```python
from build123d import *

# Parameters (mm, degrees)
SKETCH1_R           = 30
BOSS_EXTRUDE1_DEPTH = 6.35


with BuildPart() as part:
    # Sketch1 → Boss-Extrude1 (new, symmetric)
    with BuildSketch(Plane(origin=(0, 0, 0), x_dir=(0, 0, -1), z_dir=(1, 0, 0))):
        with BuildLine():
            Line((90, 0), (90, 45))
            Line((90, 45), (51.784861392, 110.303929293))
            ThreePointArc((51.784861392, 110.303929293), (0, 140), (-51.784861392, 110.303929293))
            Line((-51.784861392, 110.303929293), (-90, 45))
            Line((-90, 45), (-90, 0))
            Line((-90, 0), (90, 0))
        make_face()
        with Locations((0, 80)):
            Circle(SKETCH1_R, mode=Mode.SUBTRACT)
    extrude(amount=BOSS_EXTRUDE1_DEPTH, both=True)


solid = part.part
```
Model file for the job. Use its own axes, mm. Coordinates: 2 decimals unless noted, no trailing zeros. Order: outer loops, then holes, each group sorted by start corner. A loop starts at its lowest first (then second) coordinate and runs counter-clockwise, first axis right, second up. Notation, with made-up numbers: (13.25, 1) -> (41.25, 1) arc R15 cw to (41.25, 26) -> close; hole circle Ø8 at (81.25, 57.25). An arc over 180 degrees is marked (long way). Return JSON: item names as keys, results as strings.
Item 1: Pin check, flat tips, straight feed: P1, Ø6, axis at x = 1.5, y = 72.5, coming from the -Z side; P2, Ø1.5, axis at x = -0.5, z = -67, coming from the +Y side. Stop position of each tip, or through.
Model answer:
{"P1": "stops at z = -75.66", "P2": "stops at y = 85.59"}
Item 2: Slice it at D-D (z = -75.5). Write the cut outline in (x, y), then the cut area to 3 significant figures.
Model answer:
{"outline": "(-6.35, 0) -> (6.35, 0) -> (6.35, 69.78) -> (-6.35, 69.78) -> close", "area": "886 mm²"}
Item 3: Wall check: line 1 along Y through (x, z) = (-3.5, 0); line 2 along Y through (x, z) = (-3.25, -10.5); line 3 along Z through (x, y) = (-4.75, 92.5). Give the ranges that are in metal, low to high. Write a range as from..to.
Model answer:
{"line 1": "y = 0..50, 110..140", "line 2": "y = 0..51.9, 108.1..139.07", "line 3": "z = -62.2..-27.27, 27.27..62.2"}
Item 4: Slice it at C-C (x = -3). Write the cut outline in (y, z), then the cut area to 3 significant figures.
Model answer:
{"outline": "(0, -90) -> (45, -90) -> (110.3, -51.78) arc R60 ccw to (110.3, 51.78) -> (45, 90) -> (0, 90) -> close; hole circle Ø60 at (80, 0)", "area": "16,700 mm²"}
Item 5: Mould opens along Y. For faces 1 (the face through (-0.089, 109.745, 3.905)), 2 (the face through (6.35, 40, 1)), 3 (the face through (0.089, 139.994, -0.875)) say: pulls with the +Y half, pulls with the -Y half, needs draft (parallel to the pull), parting line crosses it, or undercut.
Model answer:
{"face 1": "undercut", "face 2": "needs draft", "face 3": "pulls with the +Y half"}
Item 6: Slice it at B-B (y = 80). Write the cut outline in (x, z), then the cut area to 3 significant figures.
Model answer:
{"outline": "(-6.35, -69.52) -> (6.35, -69.52) -> (6.35, -30) -> (-6.35, -30) -> close; (-6.35, 30) -> (6.35, 30) -> (6.35, 69.52) -> (-6.35, 69.52) -> close", "area": "1,000 mm²"}
Item 7: Slice it at A-A (z = 0). Write the cut outline in (x, y).
Model answer:
{"outline": "(-6.35, 0) -> (6.35, 0) -> (6.35, 50) -> (-6.35, 50) -> close; (-6.35, 110) -> (6.35, 110) -> (6.35, 140) -> (-6.35, 140) -> close"}
